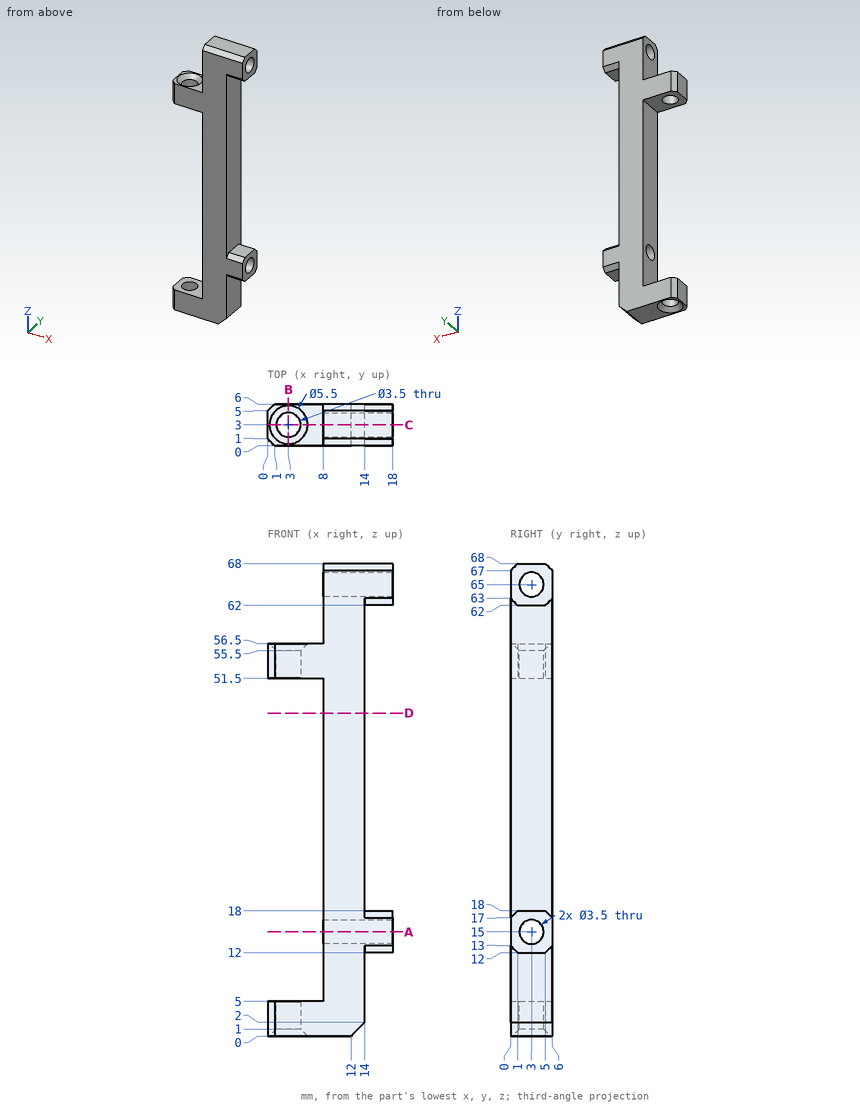
Answer from the drawing. Dimensions are ordinates in mm from the lowest x, y and z of the part. Give positions to 0.01 mm unless a question says otherwise; leave off trailing zeros. Write each loop counter-clockwise with the first axis right and the second up, starting at its lowest first coordinate (ties: lowest second). Pieces come first, ordered by that corner, then holes. Notation, with made-up numbers: (86, 22.25) -> (124, 22.25) arc R21 cw to (124, 47.25) -> close; hole circle Ø6 at (36, 68). An arc over 180 degrees is marked (long way). One line per question, with ' | ' between items. Start each with the question number.
1. Section D-D (z = 46.5) is taken. Determine the outline of the cut face in (x, y).
2. Section C-C (y = 3) is taken. State how many separate pieces and enclosed holes the cut face has, plus the area to 3 significant figures.
3. Section B-B (x = 3) is taken. Determine the outline of the cut face in (y, z).
4. Given pin 1 Ø3 at (y, z) = (5, 16.5) entering from -X; pin 2 Ø1.8 at (x, y) = (3.5, 3.5) entering from -Z; pin 3 Ø1.2 at (x, y) = (15.5, 2.5) entering from -Z; pin 4 Ø3 at (y, z) = (3, 20) entering from +X, each flat-ended and moving along its own axis, determine where each tip first touches the part or whether it passes through.
5. Section A-A (z = 15) is taken. Determine the outline of the cut face in (x, y), plus the area to 3 significant figures.
6. Find the intervals of material crossed by probe 1 along Z at (x, y) = (7.5, 3.5); probe 2 along Z at (x, y) = (12, 1.5); probe 3 along Z at (x, y) = (15.25, 4.25), in increasing order.
Response values:
1) outline: (8, 0) -> (14, 0) -> (14, 6) -> (8, 6) -> close
2) separate pieces: 5 | enclosed holes: 0 | area: 427 mm2
3) outline: (0, 0) -> (0.25, 0) -> (1.25, 1) -> (1.25, 5) -> (0, 5) -> close; (0, 51.5) -> (1.25, 51.5) -> (1.25, 55.5) -> (0.25, 56.5) -> (0, 56.5) -> close; (4.75, 1) -> (5.75, 0) -> (6, 0) -> (6, 5) -> (4.75, 5) -> close; (4.75, 51.5) -> (6, 51.5) -> (6, 56.5) -> (5.75, 56.5) -> (4.75, 55.5) -> close
4) pin 1: x = 8 | pin 2: through | pin 3: z = 12 | pin 4: x = 14
5) outline: (8, 0) -> (18, 0) -> (18, 1.25) -> (8, 1.25) -> close; (8, 4.75) -> (18, 4.75) -> (18, 6) -> (8, 6) -> close | area: 25.0 mm2
6) probe 1: 0 to 5, 51.5 to 56.5 | probe 2: 0 to 14.1, 15.9 to 64.1, 65.9 to 68 | probe 3: 12 to 13.78, 16.22 to 18, 62 to 63.78, 66.22 to 68
